Verification items for the finished model (mm, model axes). A direction names the side the tool comes from. Round coordinates to 2 decimals unless told otherwise and drop trailing zeros. Loops run counter-clockwise (first coordinate to the right, second up) from the corner with the lowest first, then second, coordinate; pieces in that order, holes last.
from build123d import *

# Parameters (mm, degrees)
SKETCH1_R           = 13.75
BOSS_EXTRUDE1_DEPTH = 2
BOSS_EXTRUDE2_DEPTH = 4
SKETCH3_R           = 14.875
CUT_EXTRUDE1_DEPTH  = 2.75
SKETCH4_R           = 12.5
CUT_EXTRUDE2_DEPTH  = 1.75
SKETCH5_R           = 8.875
BOSS_EXTRUDE3_DEPTH = 5.5
SKETCH6_R           = 6.8
CUT_EXTRUDE3_DEPTH  = 5.5


with BuildPart() as part:
    # Sketch1 → Boss-Extrude1 (new body)
    with BuildSketch(Plane(origin=(0, 0, 0), x_dir=(1, 0, 0), z_dir=(0, 1, 0))):
        Circle(SKETCH1_R)
    extrude(amount=BOSS_EXTRUDE1_DEPTH)

    # Sketch2 → Boss-Extrude2 (add)
    with BuildSketch(Plane(origin=(0, 2, 0), x_dir=(1, 0, 0), z_dir=(0, 1, 0))):
        Polygon((16.778956996, -5.710769223), (15.902637917, 7.82639063), (5.710769223, 16.778956996), (-7.82639063, 15.902637917), (-16.778956996, 5.710769223), (-15.902637917, -7.82639063), (-5.710769223, -16.778956996), (7.82639063, -15.902637917), align=None)
    extrude(amount=BOSS_EXTRUDE2_DEPTH)

    # Sketch3 → Cut-Extrude1 (cut)
    with BuildSketch(Plane(origin=(0, 6, 0), x_dir=(1, 0, 0), z_dir=(0, 1, 0))):
        Circle(SKETCH3_R)
    extrude(amount=-CUT_EXTRUDE1_DEPTH, mode=Mode.SUBTRACT)

    # Sketch4 → Cut-Extrude2 (cut)
    with BuildSketch(Plane(origin=(0, 3.25, 0), x_dir=(1, 0, 0), z_dir=(0, 1, 0))):
        Circle(SKETCH4_R)
    extrude(amount=-CUT_EXTRUDE2_DEPTH, mode=Mode.SUBTRACT)

    # Sketch5 → Boss-Extrude3 (add)
    with BuildSketch(Plane(origin=(0, 1.5, 0), x_dir=(1, 0, 0), z_dir=(0, 1, 0))):
        Circle(SKETCH5_R)
    extrude(amount=BOSS_EXTRUDE3_DEPTH)

    # Sketch6 → Cut-Extrude3 (cut)
    with BuildSketch(Plane(origin=(0, 7, 0), x_dir=(1, 0, 0), z_dir=(0, 1, 0))):
        Circle(SKETCH6_R)
    extrude(amount=-CUT_EXTRUDE3_DEPTH, mode=Mode.SUBTRACT)


solid = part.part
1. Release check for a two-part mould opening along X. For faces 1 (the face through (-1.47, 4.29, 6.64)), 2 (the face through (0, 0, 0)), 3 (the face through (0.963, 3.972, 16.347)) record: released by +X, released by -X, zero draft, split by the parting line, or undercut.
2. Tool access check on faces 4 (the face through (2, 2, 14)), 5 (the face through (-16.347, 3.972, 0.963)), 6 (the face through (8, 4.64, -12.54)). Record the directions out of +Z, -Z, +X, -X, +Y, -Y that give a thin tool (end or side, any length) a straight path to the whole face; none if there is none.
3. Section check C-C (z = 10.5). Enter the section's corners in (x, y).
4. Section check D-D (x = -9.5). Enter the section's corners in (y, z).
5. Section check B-B (y = 5). Enter the section's corners in (x, z) (3 decimals), then the cut area to 3 significant figures.
6. Gauge pin test, flat ends, axial feed: P1, Ø4, axis at x = -6.5, y = 6, coming from the -Z side; P2, Ø2, axis at x = -9, z = 13, coming from the -Y side; P3, Ø12, axis at x = 12.5, z = 9, coming from the +Y side. Record the tip position at first contact, or that the pin passes through.
7. Section check A-A (y = 2.75). Enter the section's corners in (x, z) (3 decimals), then the cut area to 3 significant figures.
8. Scan lines: L1, parallel to Z at x = -3, y = 5.5; L2, parallel to Z at x = -8, y = 3.5 (3 decimals); L3, parallel to Z at x = 0, y = 2.15 (3 decimals). Record each from-to range of solid material in increasing order.
Taken from the geometry:
1. face 1: undercut
1. face 2: zero draft
1. face 3: released by +X
2. face 4: -Y
2. face 5: +Z, -X, +Y, -Y
2. face 6: +Y
3. outline: (-12.86, 2) - (-8.88, 2) - (-8.88, 0) - (8.88, 0) - (8.88, 2) - (12.57, 2) - (12.57, 6) - (10.54, 6) - (10.54, 3.25) - (6.78, 3.25) - (6.78, 1.5) - (-6.78, 1.5) - (-6.78, 3.25) - (-10.54, 3.25) - (-10.54, 6) - (-12.86, 6) - close
4. outline: (0, -9.94) - (2, -9.94) - (2, -14) - (6, -14) - (6, -11.45) - (3.25, -11.45) - (3.25, -8.12) - (1.5, -8.12) - (1.5, 8.12) - (3.25, 8.12) - (3.25, 11.45) - (6, 11.45) - (6, 13.45) - (2, 13.45) - (2, 9.94) - (0, 9.94) - close
5. outline: (-16.779, -5.711) - (-7.826, -15.903) - (5.711, -16.779) - (15.903, -7.826) - (16.779, 5.711) - (7.826, 15.903) - (-5.711, 16.779) - (-15.903, 7.826) - close; circle Ø17.75 at (0, 0); hole circle Ø29.75 at (0, 0); hole circle Ø13.6 at (0, 0)
5. area: 296 mm2
6. P1: stops at z = -16.12
6. P2: stops at y = 2
6. P3: stops at y = 6
7. outline: (-16.779, -5.711) - (-7.826, -15.903) - (5.711, -16.779) - (15.903, -7.826) - (16.779, 5.711) - (7.826, 15.903) - (-5.711, 16.779) - (-15.903, 7.826) - close; circle Ø17.75 at (0, 0); hole circle Ø25 at (0, 0); hole circle Ø13.6 at (0, 0)
7. area: 500 mm2
8. L1: z = -16.22 to -14.57, -8.35 to -6.1, 6.1 to 8.35, 14.57 to 16.6
8. L2: z = -15.705 to -12.541, -3.843 to 3.843, 12.541 to 14.768
8. L3: z = -16.409 to -12.5, -8.875 to -6.8, 6.8 to 8.875, 12.5 to 16.409
